Model file for the job. Use its own axes, mm. A direction names the side the tool comes from. Round coordinates to 2 decimals unless told otherwise and drop trailing zeros. Order: outer loops, then holes, each group sorted by start corner. A loop starts at its lowest first (then second) coordinate and runs counter-clockwise, first axis right, second up. Notation, with made-up numbers: (28.25, 47.5) - (42.25, 47.5) arc R14 cw to (42.25, 65.5) - close; hole circle Ø9 at (67, 3.5). An arc over 180 degrees is marked (long way). Write item = value, one per line.
```python
from build123d import *

# Parameters (mm, degrees)
SKETCH1_R           = 49
SKETCH1_R_2         = 5
BOSS_EXTRUDE1_DEPTH = 15
SKETCH2_R           = 25
BOSS_EXTRUDE2_DEPTH = 60
F_3DSKETCH1_R       = 17.5
F_3DSKETCH1_R_2     = 6
BOSS_EXTRUDE3_DEPTH = 15
SKETCH3_R           = 17.5
CUT_EXTRUDE1_DEPTH  = 60


with BuildPart() as part:
    # Sketch1 → Boss-Extrude1 (new body)
    with BuildSketch(Plane.XY):
        with Locations((2.00095732, -3.501675309)):
            Circle(SKETCH1_R)
        with Locations((2.00095732, 31.498324691)):
            Circle(SKETCH1_R_2, mode=Mode.SUBTRACT)
        with Locations((37.00095732, -3.501675309)):
            Circle(SKETCH1_R_2, mode=Mode.SUBTRACT)
        with Locations((2.00095732, -38.501675309)):
            Circle(SKETCH1_R_2, mode=Mode.SUBTRACT)
        with Locations((-32.99904268, -3.501675309)):
            Circle(SKETCH1_R_2, mode=Mode.SUBTRACT)
        with Locations((26.749694661, 21.247062032)):
            Circle(SKETCH1_R_2, mode=Mode.SUBTRACT)
        with Locations((-22.747780022, -28.250412651)):
            Circle(SKETCH1_R_2, mode=Mode.SUBTRACT)
    extrude(amount=BOSS_EXTRUDE1_DEPTH)

    # Sketch2 → Boss-Extrude2 (add)
    with BuildSketch(Plane.XY.offset(15)):
        with Locations((2.00095732, -3.501675309)):
            Circle(SKETCH2_R)
    extrude(amount=BOSS_EXTRUDE2_DEPTH)

    # 3DSketch1 → Boss-Extrude3 (add)
    with BuildSketch(Plane(origin=(17.828624009, 46.498324691, 90), x_dir=(-0.2889903749033983, -0.9573320026057801, 0), z_dir=(0, 0, -1))):
        with BuildLine():
            Line((0, 0), (33.502008681, -22.56364586))
            ThreePointArc((33.502008681, -22.56364586), (43.770932214, -28.017146975), (55.342156817, -29.156544228))
            Line((55.342156817, -29.156544228), (96.002707212, -28.719960078))
            ThreePointArc((96.002707212, -28.719960078), (114.697542875, -18.694835663), (104.672418459, 0))
            Line((104.672418459, 0), (70.251663663, 24.843392205))
            ThreePointArc((70.251663663, 24.843392205), (60.424969024, 29.620810014), (49.539130104, 30.562170435))
            Line((49.539130104, 30.562170435), (8.568124101, 28.383434594))
            ThreePointArc((8.568124101, 28.383434594), (-9.907655246, 18.475779348), (0, 0))
        make_face()
        with Locations(Location((52.440643461, 0.702813104, 0), (0, 0, 253.202479102))):
            Circle(F_3DSKETCH1_R, mode=Mode.SUBTRACT)
        with Locations(Location((100.308395753, -13.747053445, 0), (0, 0, 253.202479102))):
            Circle(F_3DSKETCH1_R_2, mode=Mode.SUBTRACT)
        with Locations(Location((4.571400625, 15.153129604, 0), (0, 0, 253.202479102))):
            Circle(F_3DSKETCH1_R_2, mode=Mode.SUBTRACT)
    extrude(amount=BOSS_EXTRUDE3_DEPTH)

    # Sketch3 → Cut-Extrude1 (cut)
    with BuildSketch(Plane.XY.offset(75)):
        with Locations((2.00095732, -3.501675309)):
            Circle(SKETCH3_R)
    extrude(amount=-CUT_EXTRUDE1_DEPTH, mode=Mode.SUBTRACT)


solid = part.part
```
1) Wall check: line 1 along Z through (x, y) = (-23, -8); line 2 along Z through (x, y) = (34, -32.5); line 3 along Z through (x, y) = (8.5, -62). Give the ranges that are in metal, low to high.
Conclusion:
line_1 = 0 to 15, 75 to 90
line_2 = 0 to 15
line_3 = 75 to 90
2) Cut at B-B (y = 24). Write the cut outline in (x, z), and give its area (3 significant figures).
Conclusion:
outline = (-38.55, 0) - (22.58, 0) - (22.58, 15) - (-38.55, 15) - close; (-19.94, 75) - (24.78, 75) - (24.78, 90) - (-19.94, 90) - close; (30.92, 0) - (42.56, 0) - (42.56, 15) - (30.92, 15) - close
area = 1,760 mm^2
3) Cut at D-D (z = 78). Write the cut outline in (x, y), and give its area (3 significant figures).
Conclusion:
outline = (-26.26, -13.58) - (-12.42, -53.71) arc R15 ccw to (17.58, -53.71) - (29.75, -14.91) arc R30 ccw to (29.75, 7.91) - (17.83, 46.5) arc R14.82 ccw to (-11.82, 46.5) - (-25.75, 7.91) arc R30 ccw to start; hole circle Ø35 at (2, -3.5); hole circle Ø12 at (2, -53.5); hole circle Ø12 at (2, 46.5)
area = 4,150 mm^2
4) 3-axis set-ups, long thin cutter, end or side, ignore diameter. For faces 1 (the face through (23.749, -34.037, 82.605)), 2 (the face through (13.5, -25.7, 44.6)), 3 (the face through (23.705, 27.472, 82.605)), 4 (the face through (18.693, -8.758, 53.025)), 5 (the face through (-18.13, -30.17, 7.4)): which of +Z, -Z, +X, -X, +Y, -Y reach the whole face in a straight line?
Conclusion:
face_1 = +Z, +X, -Y
face_2 = none
face_3 = +Z, +X, +Y
face_4 = +Z
face_5 = -Z
5) Cut at A-A (x = 25). Write the cut outline in (y, z).
Conclusion:
outline = (-46.77, 0) - (16.56, 0) - (16.56, 15) - (6.3, 15) - (6.3, 75) - (23.28, 75) - (23.28, 90) - (-30.05, 90) - (-30.05, 75) - (-13.3, 75) - (-13.3, 15) - (-46.77, 15) - close; (25.93, 0) - (39.77, 0) - (39.77, 15) - (25.93, 15) - close
6) Mould opens along X. For faces 6 (the face through (2, -3, 15)), 7 (the face through (4.308, -42.938, 7.395)), 8 (the face through (-20.5, 8.1, 15)), 9 (the face through (-27.994, -2.942, 82.605)) say: +X half, -X half, draft (parallel to the pull), parting line (faces both ways), or undercut.
Conclusion:
face_6 = undercut
face_7 = undercut
face_8 = draft
face_9 = -X half
7) Cut at C-C (z = 11.5). Write the cut outline in (x, y).
Conclusion:
outline = circle Ø98 at (2, -3.5); hole circle Ø10 at (-33, -3.5); hole circle Ø10 at (-22.75, -28.25); hole circle Ø10 at (2, -38.5); hole circle Ø10 at (2, 31.5); hole circle Ø10 at (26.75, 21.25); hole circle Ø10 at (37, -3.5)
8) Flat gauge pins, fed straight in: pin 1 Ø4 at (x, z) = (3.5, 49) entering from -Y; pin 2 Ø6 at (x, z) = (35.5, 15.5) entering from +Y; pin 3 Ø8 at (x, y) = (2, 31.5) entering from -Z; pin 4 Ø16 at (x, y) = (-22.75, -28.25) entering from +Z. Where does each tip first touch, or does it go through?
Conclusion:
pin_1 = -28.5
pin_2 = 34.82
pin_3 = 75
pin_4 = 90
